The listing builds one solid part. Answer for the finished solid, in the listing's coordinates (mm). Coordinates: 2 decimals unless noted, no trailing zeros. Write each loop counter-clockwise with the first axis right and the second up, starting at its lowest first coordinate (ties: lowest second). Pieces come first, ordered by that corner, then holes. Notation, with made-up numbers: M 45,67.5 L 73,67.5 A32 cw 73,96.5 Z; hole C -13.75,-37.75 d7. An arc over 180 degrees is marked long. Answer as CSV lines item,"result".
Autodesk Inventor part; units mm, degrees
ref_plane "YZ Plane" through (0, 0, 0) normal (1, 0, 0) x (0, 1, 0)
ref_plane "XZ Plane" through (0, 0, 0) normal (0, 1, 0) x (-1, 0, 0)
ref_plane "XY Plane" through (0, 0, 0) normal (0, 0, 1) x (1, 0, 0)
sketch "Skizze1" plane through (0, 0, 0) normal (0, 1, 0) x (-1, 0, 0)
  line L0 (0, 0) -> (-655, 0)
  line L1 (-655, 0) -> (-655, 200)
  line L2 (-655, 200) -> (0, 200)
  line L3 (0, 200) -> (0, 0)
  line L4 (-327.5, 0) -> (-327.5, 200) construction
  line L5 (0, 100) -> (-655, 100) construction
  line L6 (-655, 55) -> (0, 55) construction
  line L7 (0, 80) -> (-655, 80) construction
  line L8 (-640, 185) -> (-640, 15) construction
  line L9 (-640, 15) -> (-15, 15) construction
  line L10 (-15, 15) -> (-15, 185) construction
  line L11 (-15, 185) -> (-640, 185) construction
  circle A0 centre (-15, 47.5) radius 3.25
  circle A1 centre (-15, 62.5) radius 3.25
  circle A2 centre (-320, 185) radius 3.25
  circle A3 centre (-335, 185) radius 3.25
  circle A4 centre (-640, 47.5) radius 3.25
  circle A5 centre (-640, 62.5) radius 3.25
  line L12 (-90, 200) -> (-90, 190)
  line L13 (-90, 190) -> (-10, 110)
  line L14 (-10, 110) -> (0, 110)
  line L15 (-565, 200) -> (-565, 190)
  line L16 (-565, 190) -> (-645, 110)
  line L17 (-645, 110) -> (-655, 110)
  circle A6 centre (-70, 130) radius 15
  circle A7 centre (-70, 40) radius 15
  circle A8 centre (-585, 130) radius 15
  circle A9 centre (-585, 40) radius 15
  point P0 (-15, 55)
  point P1 (-327.5, 185)
  point P2 (-565, 200)
  point P3 (-655, 110)
  dimension "d0" = 655
  dimension "d1" = 200
  dimension "d2" = 145
  dimension "d3" = 80
  dimension "d6" = 15
  dimension "d13" = 6.5
  dimension "d14" = 7.5
  dimension "d21" = 6.5
  dimension "d23" = 7.5
  dimension "d80" = 625
  dimension "d81" = 45
  dimension "d83" = 90
  dimension "d84" = 90
  dimension "d85" = 10
  dimension "d86" = 30
  dimension "d87" = 70
  dimension "d88" = 70
  dimension "d91" = 90
extrude "Ex-Platte" add sketch "Skizze1" along normal blind 3 contours L0 L1 L17 L16 L15 L2 L12 L13 L14 L3
sketch "S-Anschraubpunkte" plane through (0, 0, 0) normal (0, 1, 0) x (-1, 0, 0)
  line L0 (-655, 0) -> (0, 0) construction
  line L1 (-90, 200) -> (-565, 200) construction
  line L2 (-655, 0) -> (0, 0) construction
  line L3 (-327.5, 0) -> (-327.5, 200) construction
  line L4 (-129.8577, 12.8998) -> (-226.8577, 12.8998) construction
  line L5 (-226.8577, 12.8998) -> (-226.8577, 171.8998) construction
  line L6 (-226.8577, 171.8998) -> (-129.8577, 171.8998) construction
  line L7 (-129.8577, 171.8998) -> (-129.8577, 12.8998) construction
  line L8 (-272.665, 68.869) -> (-382.335, 68.869) construction
  line L9 (-382.335, 68.869) -> (-382.335, 153.169) construction
  line L10 (-382.335, 153.169) -> (-272.665, 153.169) construction
  line L11 (-272.665, 153.169) -> (-272.665, 68.869) construction
  line L12 (-463.0213, 68.519) -> (-519.0213, 68.519) construction
  line L13 (-519.0213, 68.519) -> (-519.0213, 153.519) construction
  line L14 (-519.0213, 153.519) -> (-463.0213, 153.519) construction
  line L15 (-463.0213, 153.519) -> (-463.0213, 68.519) construction
  line L16 (-491.0213, 68.519) -> (-491.0213, 153.519) construction
  line L17 (-463.0213, 111.019) -> (-519.0213, 111.019) construction
  line L18 (-327.5, 68.869) -> (-327.5, 153.169) construction
  line L19 (-272.665, 111.019) -> (-382.335, 111.019) construction
  line L20 (-178.3577, 12.8998) -> (-178.3577, 171.8998) construction
  line L21 (-226.8577, 92.3998) -> (-129.8577, 92.3998) construction
  circle A0 centre (-466.5213, 150.019) radius 1.35
  circle A1 centre (-448.0213, 68.519) radius 2.15
  circle A2 centre (-463.0213, 53.519) radius 2.15
  circle A3 centre (-534.0213, 68.519) radius 2.15
  circle A4 centre (-519.0213, 53.519) radius 2.15
  circle A5 centre (-448.0213, 153.519) radius 2.15
  circle A6 centre (-463.0213, 168.519) radius 2.15
  circle A7 centre (-519.0213, 168.519) radius 2.15
  circle A8 centre (-534.0213, 153.519) radius 2.15
  circle A9 centre (-276.645, 149.169) radius 1.65
  circle A10 centre (-276.645, 73.069) radius 1.65
  circle A11 centre (-377.995, 73.069) radius 1.65
  circle A12 centre (-377.995, 149.169) radius 1.65
  circle A13 centre (-257.665, 153.169) radius 2.15
  circle A14 centre (-272.665, 168.169) radius 2.15
  circle A15 centre (-257.665, 68.869) radius 2.15
  circle A16 centre (-272.665, 53.869) radius 2.15
  circle A17 centre (-397.335, 153.169) radius 2.15
  circle A18 centre (-382.335, 168.169) radius 2.15
  circle A19 centre (-382.335, 53.869) radius 2.15
  circle A20 centre (-397.335, 68.869) radius 2.15
  circle A21 centre (-178.3577, 122.1498) radius 1.65
  circle A22 centre (-178.3577, 57.1498) radius 1.65
  circle A23 centre (-515.5213, 150.019) radius 1.35
  circle A24 centre (-466.5213, 92.019) radius 1.35
  circle A25 centre (-515.5213, 92.019) radius 1.35
  circle A26 centre (-422.6782, 165) radius 2.15
  circle A27 centre (-422.6782, 180) radius 2.15
  line L22 (-422.6782, 165) -> (-422.6782, 180) construction
  circle A28 centre (-560.7476, 111.019) radius 2.15
  circle A29 centre (-545.7476, 111.019) radius 2.15
  line L23 (-560.7476, 111.019) -> (-545.7476, 111.019) construction
  circle A30 centre (-297.5, 25.1204) radius 2.15
  circle A31 centre (-312.5, 25.1204) radius 2.15
  line L24 (-297.5, 25.1204) -> (-312.5, 25.1204) construction
  circle A32 centre (-342.5, 25.1204) radius 2.15
  circle A33 centre (-357.5, 25.1204) radius 2.15
  line L25 (-342.5, 25.1204) -> (-357.5, 25.1204) construction
  circle A34 centre (-498.5213, 37.836) radius 2.15
  circle A35 centre (-483.5213, 37.836) radius 2.15
  line L26 (-498.5213, 37.836) -> (-483.5213, 37.836) construction
  circle A36 centre (-422.6782, 103.519) radius 2.15
  circle A37 centre (-422.6782, 118.519) radius 2.15
  line L27 (-422.6782, 103.519) -> (-422.6782, 118.519) construction
  line L28 (-312.5, 25.1204) -> (-342.5, 25.1204) construction
  point P0 (-422.6782, 111.019)
  point P1 (-491.0213, 37.836)
  point P2 (-327.5, 25.1204)
  dimension "d96" = 97
  dimension "d97" = 159
  dimension "d98" = 109.67
  dimension "d99" = 84.3
  dimension "d100" = 56
  dimension "d101" = 85
  dimension "d102" = 2.7
  dimension "d105" = 4.3
  dimension "d106" = 4.3
  dimension "d107" = 15
  dimension "d108" = 15
  dimension "d110" = 3.98
  dimension "d111" = 3.3
  dimension "d112" = 4
  dimension "d115" = 76.1
  dimension "d122" = 101.35
  dimension "d127" = 4.3
  dimension "d128" = 4.3
  dimension "d129" = 15
  dimension "d130" = 15
  dimension "d132" = 49.75
  dimension "d135" = 65
  dimension "d140" = 3.3
  dimension "d154" = 3.5
  dimension "d155" = 3.5
  dimension "d158" = 58
  dimension "d174" = 4.3
  dimension "d176" = 4.3
  dimension "d177" = 15
  dimension "d178" = 20
  dimension "d195" = 4.3
  dimension "d196" = 4.3
  dimension "d197" = 15
  dimension "d214" = 4.3
  dimension "d215" = 4.3
  dimension "d216" = 15
  dimension "d233" = 4.3
  dimension "d234" = 4.3
  dimension "d235" = 15
  dimension "d252" = 4.3
  dimension "d253" = 4.3
  dimension "d254" = 15
  dimension "d271" = 4.3
  dimension "d272" = 4.3
  dimension "d273" = 15
  dimension "d274" = 30
extrude "Ex-Anschraubpunkte" cut sketch "S-Anschraubpunkte" along normal blind 3
chamfer "Fase-5mm" distance 5 angle 45 6 edges at (655, 1.5, 0) (0, 1.5, 0) (0, 1.5, 110) (90, 1.5, 200) (565, 1.5, 200) (655, 1.5, 110)
equation "\"d21\" = d13"
equation "\"d23\" = d14"
equation "\"d84\" = d83"
properties part number "enc-ElectronicsPanel V1"
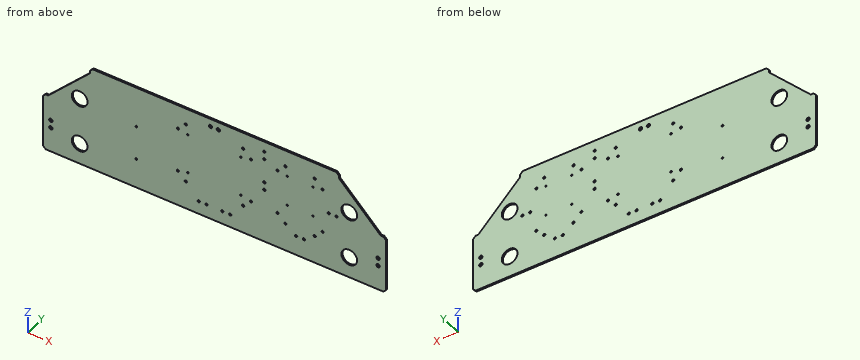
Q1. Straight lines are drawn through the part: line 1 (Z direction, x = 15, y = 1.5); line 2 (X direction, y = 2.6, z = 37); line 3 (X direction, y = 1.95, z = 122.5). For each, find the intervals that lie inside material, in ascending order.
Output:
line 1,"0 to 44.25, 50.75 to 59.25, 65.75 to 115"
line 2,"0 to 55.3, 84.7 to 481.54, 485.5 to 496.54, 500.5 to 570.3, 599.7 to 655"
line 3,"22.5 to 57.01, 82.99 to 176.75, 179.97 to 572.01, 597.99 to 632.5"
Q2. Flat-ended cylindrical pins translate along their axes: pin 1 Ø4 at (x, z) = (397.335, 68.869) entering from +Y; pin 2 Ø5.5 at (x, z) = (382.335, 53.869) entering from +Y. Find the tip coordinate at first contact, or state that the pin passes through.
Output:
pin 1,"through"
pin 2,"y = 3"
Q3. Find section A-A (z = 130). Give the vertices of the cut face in (x, y), and give its area (4 significant figures).
Output:
outline,"M 30,0 L 55,0 L 55,3 L 30,3 Z; M 85,0 L 570,0 L 570,3 L 85,3 Z; M 600,0 L 625,0 L 625,3 L 600,3 Z"
area,"1,605 mm2"
Q4. Find section C-C (y = 0.95). Count the separate pieces of the cut face and the enclosed holes in it, and give its area (3 significant figures).
Output:
separate pieces,"1"
enclosed holes,"48"
area,"118,000 mm2"
Q5. Find section B-B (x = 585). Give the vertices of the cut face in (y, z), and give its area (3 significant figures).
Output:
outline,"M 0,0 L 3,0 L 3,25 L 0,25 Z; M 0,55 L 3,55 L 3,115 L 0,115 Z; M 0,145 L 3,145 L 3,170 L 0,170 Z"
area,"330 mm2"
